Geometry check sheet. Reference: the model listing, model coordinates, mm. Coordinates: 2 decimals unless noted, no trailing zeros. Write each loop counter-clockwise with the first axis right and the second up, starting at its lowest first coordinate (ties: lowest second). Pieces come first, ordered by that corner, then holes. Notation, with made-up numbers: (85, -6) -> (144, -6) arc R19 cw to (144, 24) -> close; hole circle Ø7 at (-16, 84). An arc over 180 degrees is marked (long way). Answer in a Markdown table with one row per item. Add a question column.
1. Cross-section at B-B on x = 0. Give the number of separate pieces and of enclosed holes in the cut face, and give its area (3 significant figures).
2. Cross-section at C-C on z = 25.5. Record the cut outline in (x, y), and give its area (3 significant figures).
3. Scan lines: L1, parallel to Z at x = -0.25, y = 3.25; L2, parallel to Y at x = -5, z = 22; L3, parallel to X at y = -2.25, z = 63.4. Record each from-to range of solid material in increasing order. Write a range as from..to.
4. Depth check by flat-ended pin: P1, Ø3, axis at x = 0, z = 13.4, coming from the -Y side; P2, Ø5, axis at x = 0, z = 88.4, coming from the +Y side; P3, Ø0.5, axis at y = 1.5, z = 49.5, coming from the +X side. Enter the tip coordinate at first touch or a pass-through.
5. Cross-section at A-A on z = 88.4. Record the cut outline in (x, y), and give its area (3 significant figures).
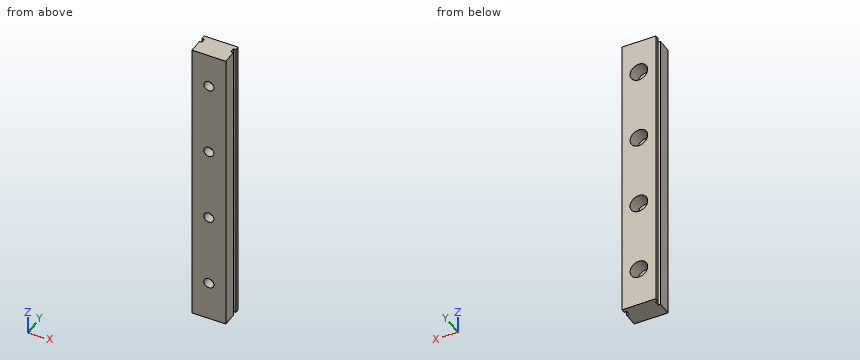
```python
from build123d import *

# Parameters (mm, degrees)
SKETCH1_W           = 11.5
SKETCH1_H           = 7.8
BOSS_EXTRUDE1_DEPTH = 100
SKETCH2_W           = 0.835250229
SKETCH2_H           = 1.6
CUT_EXTRUDE1_DEPTH  = 101.241071922
SKETCH3_R           = 3
CUT_EXTRUDE2_DEPTH  = 4.7
SKETCH4_R           = 1.7
CUT_EXTRUDE3_DEPTH  = 101.27538332


with BuildPart() as part:
    # Sketch1 → Boss-Extrude1 (new body)
    with BuildSketch(Plane.XY):
        Rectangle(SKETCH1_W, SKETCH1_H)
    extrude(amount=BOSS_EXTRUDE1_DEPTH)

    # Sketch2 → Cut-Extrude1 (cut, through all)
    with BuildSketch(Plane.XY.offset(100)):
        with Locations((5.332374886, 1.7)):
            Rectangle(SKETCH2_W, SKETCH2_H)
        with Locations((-5.332374886, 1.7)):
            Rectangle(SKETCH2_W, SKETCH2_H)
    extrude(amount=-CUT_EXTRUDE1_DEPTH, mode=Mode.SUBTRACT)

    # Sketch3 → Cut-Extrude2 (cut)
    with BuildSketch(Plane(origin=(0, 3.9, 0), x_dir=(1, 0, 0), z_dir=(0, 1, 0))):
        with Locations(Location((0, -88.4, 0), (0, 0, 270))):
            Circle(SKETCH3_R)
        with Locations(Location((0, -63.4, 0), (0, 0, 270))):
            Circle(SKETCH3_R)
        with Locations(Location((0, -38.4, 0), (0, 0, 270))):
            Circle(SKETCH3_R)
        with Locations(Location((0, -13.4, 0), (0, 0, 270))):
            Circle(SKETCH3_R)
        with Locations((0, 11.6)):
            Circle(SKETCH3_R)
        with Locations((0, 36.6)):
            Circle(SKETCH3_R)
        with Locations((0, 61.6)):
            Circle(SKETCH3_R)
        with Locations((0, 86.6)):
            Circle(SKETCH3_R)
        with Locations((0, 111.6)):
            Circle(SKETCH3_R)
        with Locations((0, 136.6)):
            Circle(SKETCH3_R)
        with Locations((0, 161.6)):
            Circle(SKETCH3_R)
        with Locations((0, 186.6)):
            Circle(SKETCH3_R)
        with Locations((0, 211.6)):
            Circle(SKETCH3_R)
        with Locations((0, 236.6)):
            Circle(SKETCH3_R)
        with Locations((0, 261.6)):
            Circle(SKETCH3_R)
        with Locations((0, 286.6)):
            Circle(SKETCH3_R)
        with Locations((0, 311.6)):
            Circle(SKETCH3_R)
        with Locations((0, 336.6)):
            Circle(SKETCH3_R)
        with Locations((0, 361.6)):
            Circle(SKETCH3_R)
        with Locations((0, 386.6)):
            Circle(SKETCH3_R)
        with Locations((0, 411.6)):
            Circle(SKETCH3_R)
        with Locations((0, 436.6)):
            Circle(SKETCH3_R)
        with Locations((0, 461.6)):
            Circle(SKETCH3_R)
        with Locations((0, 486.6)):
            Circle(SKETCH3_R)
        with Locations((0, 511.6)):
            Circle(SKETCH3_R)
    extrude(amount=-CUT_EXTRUDE2_DEPTH, mode=Mode.SUBTRACT)

    # Sketch4 → Cut-Extrude3 (cut, through all)
    with BuildSketch(Plane(origin=(0, -0.8, 0), x_dir=(1, 0, 0), z_dir=(0, 1, 0))):
        with Locations(Location((0, -88.4, 0), (0, 0, 270))):
            Circle(SKETCH4_R)
        with Locations(Location((0, -63.4, 0), (0, 0, 270))):
            Circle(SKETCH4_R)
        with Locations(Location((0, -38.4, 0), (0, 0, 270))):
            Circle(SKETCH4_R)
        with Locations(Location((0, -13.4, 0), (0, 0, 270))):
            Circle(SKETCH4_R)
        with Locations((0, 11.6)):
            Circle(SKETCH4_R)
        with Locations((0, 36.6)):
            Circle(SKETCH4_R)
        with Locations((0, 61.6)):
            Circle(SKETCH4_R)
        with Locations((0, 86.6)):
            Circle(SKETCH4_R)
        with Locations((0, 111.6)):
            Circle(SKETCH4_R)
        with Locations((0, 136.6)):
            Circle(SKETCH4_R)
        with Locations((0, 161.6)):
            Circle(SKETCH4_R)
        with Locations((0, 186.6)):
            Circle(SKETCH4_R)
        with Locations((0, 211.6)):
            Circle(SKETCH4_R)
        with Locations((0, 236.6)):
            Circle(SKETCH4_R)
        with Locations((0, 261.6)):
            Circle(SKETCH4_R)
        with Locations((0, 286.6)):
            Circle(SKETCH4_R)
        with Locations((0, 311.6)):
            Circle(SKETCH4_R)
        with Locations((0, 336.6)):
            Circle(SKETCH4_R)
        with Locations((0, 361.6)):
            Circle(SKETCH4_R)
        with Locations((0, 386.6)):
            Circle(SKETCH4_R)
        with Locations((0, 411.6)):
            Circle(SKETCH4_R)
        with Locations((0, 436.6)):
            Circle(SKETCH4_R)
        with Locations((0, 461.6)):
            Circle(SKETCH4_R)
        with Locations((0, 486.6)):
            Circle(SKETCH4_R)
        with Locations((0, 511.6)):
            Circle(SKETCH4_R)
    extrude(amount=-CUT_EXTRUDE3_DEPTH, mode=Mode.SUBTRACT)


solid = part.part
```
Results found:
| question | item | result |
|---|---|---|
| 1 | separate pieces | 5 |
| 1 | enclosed holes | 0 |
| 1 | area | 625 mm^2 |
| 2 | outline | (-5.75, -3.9) -> (5.75, -3.9) -> (5.75, 0.9) -> (4.91, 0.9) -> (4.91, 2.5) -> (5.75, 2.5) -> (5.75, 3.9) -> (-5.75, 3.9) -> (-5.75, 2.5) -> (-4.91, 2.5) -> (-4.91, 0.9) -> (-5.75, 0.9) -> close |
| 2 | area | 87.0 mm^2 |
| 3 | L1 | z = 0..10.41, 16.39..35.41, 41.39..60.41, 66.39..85.41, 91.39..100 |
| 3 | L2 | y = -3.9..0.9, 2.5..3.9 |
| 3 | L3 | x = -5.75..-1.7, 1.7..5.75 |
| 4 | P1 | passes through |
| 4 | P2 | stops at y = -0.8 |
| 4 | P3 | stops at x = 4.91 |
| 5 | outline | (-5.75, -3.9) -> (-1.7, -3.9) -> (-1.7, -0.8) -> (-3, -0.8) -> (-3, 3.9) -> (-5.75, 3.9) -> (-5.75, 2.5) -> (-4.91, 2.5) -> (-4.91, 0.9) -> (-5.75, 0.9) -> close; (1.7, -3.9) -> (5.75, -3.9) -> (5.75, 0.9) -> (4.91, 0.9) -> (4.91, 2.5) -> (5.75, 2.5) -> (5.75, 3.9) -> (3, 3.9) -> (3, -0.8) -> (1.7, -0.8) -> close |
| 5 | area | 48.3 mm^2 |
